Check sheet for the drawn part. Datum: minimum x, y, z corner. Units: mm. A direction names the side the tool comes from. Coordinates: 2 decimals unless noted, no trailing zeros. Write each loop counter-clockwise with the first axis right and the second up, starting at its lowest first coordinate (ties: lowest second). Pieces come first, ordered by that corner, then holes. Notation, with made-up numbers: (5.5, 50.25) -> (48.5, 50.25) arc R12 cw to (48.5, 72.25) -> close; hole circle Ø5 at (-37, 46). An arc over 180 degrees is marked (long way). Write item = value, one per line. Start each with the question number.
(1) Section check D-D (x = 147). Record the cut outline in (y, z), plus the area to 3 significant figures.
(2) Gauge pin test, flat ends, axial feed: pin 1 Ø7 at (y, z) = (5.5, 151) entering from -X; pin 2 Ø4 at (x, z) = (167.56, 38.1) entering from -Y; pin 3 Ø8 at (x, y) = (120, 5.5) entering from -Z; pin 4 Ø4 at (x, z) = (160, 149.5) entering from -Y. Record the tip position at first contact, or that the pin passes through.
(3) Section check C-C (x = 185). Record the cut outline in (y, z), plus the area to 3 significant figures.
(4) Section check B-B (z = 85). Record the cut outline in (x, y).
(5) Section check A-A (y = 6.75). Record the cut outline in (x, z), plus the area to 3 significant figures.
(6) Set-up check for the marked faces 1, 2 and 3: record each of +Z, -Z, +X, -X, +Y, -Y from which the full face is reachable in a straight line by a thin tool's end or side.
(7) Material ranges on probe 1 along X at (y, z) = (23.4, 38.1); probe 2 along X at (y, z) = (8.25, 93); probe 3 along Z at (x, y) = (177.72, 23.5), recorded low to high. Write a range as [from, to].
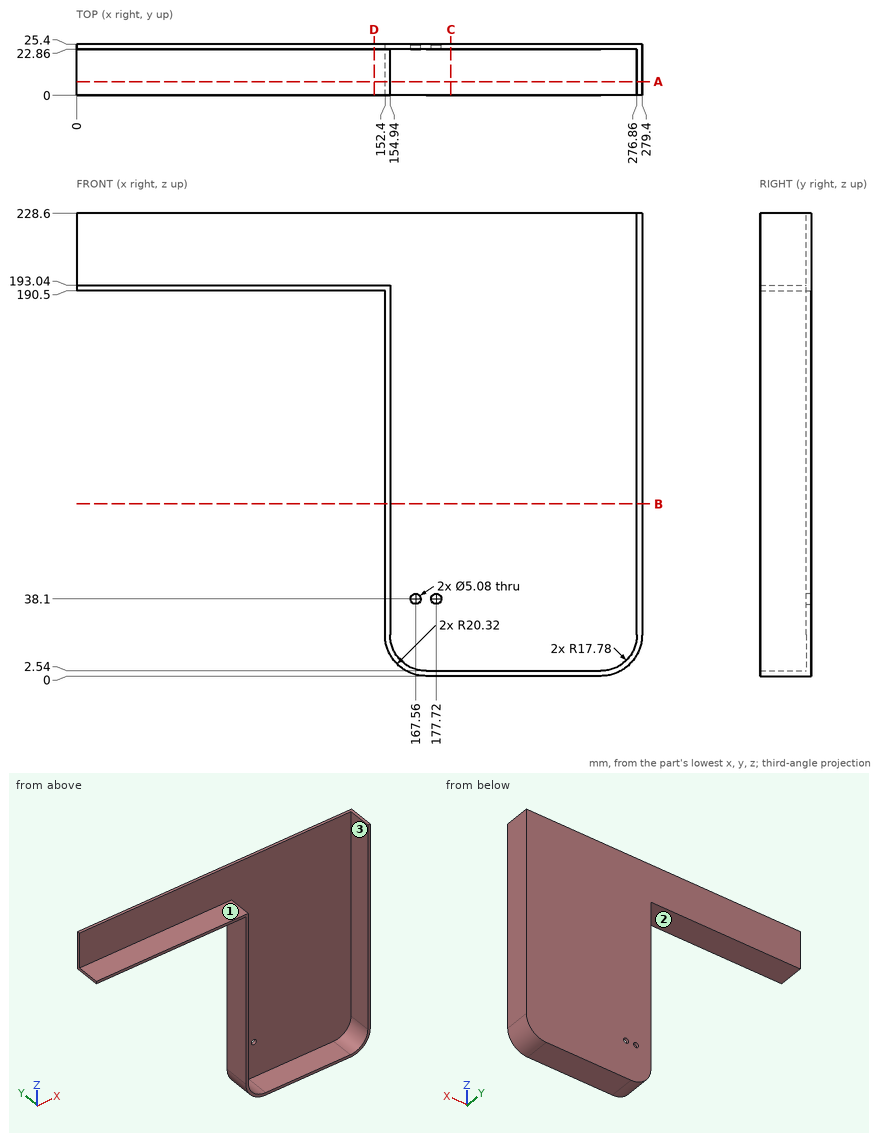
Response:
q1.outline = (0, 190.5) -> (25.4, 190.5) -> (25.4, 228.6) -> (22.86, 228.6) -> (22.86, 193.04) -> (0, 193.04) -> close
q1.area = 155 mm2
q2.pin_1 = 152.4
q2.pin_2 = through
q2.pin_3 = 190.5
q2.pin_4 = 22.86
q3.outline = (0, 0) -> (25.4, 0) -> (25.4, 228.6) -> (22.86, 228.6) -> (22.86, 2.54) -> (0, 2.54) -> close
q3.area = 639 mm2
q4.outline = (152.4, 0) -> (154.94, 0) -> (154.94, 22.86) -> (276.86, 22.86) -> (276.86, 0) -> (279.4, 0) -> (279.4, 25.4) -> (152.4, 25.4) -> close
q5.outline = (0, 190.5) -> (152.4, 190.5) -> (152.4, 20.32) arc R20.32 ccw to (172.72, 0) -> (259.08, 0) arc R20.32 ccw to (279.4, 20.32) -> (279.4, 228.6) -> (276.86, 228.6) -> (276.86, 20.32) arc R17.78 cw to (259.08, 2.54) -> (172.72, 2.54) arc R17.78 cw to (154.94, 20.32) -> (154.94, 193.04) -> (0, 193.04) -> close
q5.area = 1,730 mm2
q6.face_1 = +Z, -X, -Y
q6.face_2 = -Z, -X, +Y, -Y
q6.face_3 = +Z, -Y
q7.probe_1 = [152.4, 165.02], [170.1, 175.18], [180.26, 279.4]
q7.probe_2 = [152.4, 154.94], [276.86, 279.4]
q7.probe_3 = [0, 35.56], [40.64, 228.6]
